Read the model definition and answer for the solid it produces. Units are mm, in the model's axes. A direction names the side the tool comes from. Give positions to 0.01 mm unless a question says otherwise; leave off trailing zeros. Write each loop counter-clockwise with the first axis right and the second up, starting at its lowest first coordinate (ties: lowest second). Pieces come first, ordered by that corner, then holes. Notation, with made-up numbers: (-12, -30) -> (-5, -30) arc R17 ccw to (-5, -5) -> close; hole circle Ø9 at (-12, -37). An arc over 180 degrees is marked (long way). Write item = value, one per line.
from build123d import *

# Parameters (mm, degrees)
SKETCH1_W           = 82.927984002
SKETCH1_H           = 60.776462656
BOSS_EXTRUDE1_DEPTH = 2
SKETCH2_W           = 82.927984002
SKETCH2_H           = 1.944543981
BOSS_EXTRUDE2_DEPTH = 55
SKETCH3_W           = 82.927984002
SKETCH3_H           = 1.52283727
BOSS_EXTRUDE3_DEPTH = 55
SKETCH4_W           = 1.238263506
SKETCH4_H           = 57.309081405
BOSS_EXTRUDE4_DEPTH = 55
SKETCH5_W           = 55
SKETCH5_H           = 1.968247646
BOSS_EXTRUDE5_DEPTH = 59
SKETCH6_W           = 41.500434797
SKETCH6_H           = 30.602093287
CUT_EXTRUDE1_DEPTH  = 59


with BuildPart() as part:
    # Sketch1 → Boss-Extrude1 (new body)
    with BuildSketch(Plane(origin=(0, 0, 0), x_dir=(0, 0, -1), z_dir=(1, 0, 0))):
        with Locations((-67.649308223, 21.107365524)):
            Rectangle(SKETCH1_W, SKETCH1_H)
    extrude(amount=BOSS_EXTRUDE1_DEPTH)

    # Sketch2 → Boss-Extrude2 (add)
    with BuildSketch(Plane(origin=(2, 0, 0), x_dir=(0, 0, -1), z_dir=(1, 0, 0))):
        with Locations((-67.649308223, 50.523324862)):
            Rectangle(SKETCH2_W, SKETCH2_H)
    extrude(amount=BOSS_EXTRUDE2_DEPTH)

    # Sketch3 → Boss-Extrude3 (add)
    with BuildSketch(Plane(origin=(2, 0, 0), x_dir=(0, 0, -1), z_dir=(1, 0, 0))):
        with Locations((-67.649308223, -8.519447169)):
            Rectangle(SKETCH3_W, SKETCH3_H)
    extrude(amount=BOSS_EXTRUDE3_DEPTH)

    # Sketch4 → Boss-Extrude4 (add)
    with BuildSketch(Plane(origin=(2, 0, 0), x_dir=(0, 0, -1), z_dir=(1, 0, 0))):
        with Locations((-108.494168471, 20.896512169)):
            Rectangle(SKETCH4_W, SKETCH4_H)
    extrude(amount=BOSS_EXTRUDE4_DEPTH)

    # Sketch5 → Boss-Extrude5 (add)
    with BuildSketch(Plane(origin=(0, 49.551052871, 0), x_dir=(-1, 0, 0), z_dir=(0, -1, 0))):
        with Locations((-29.5, -27.169440045)):
            Rectangle(SKETCH5_W, SKETCH5_H)
    extrude(amount=BOSS_EXTRUDE5_DEPTH)

    # Sketch6 → Cut-Extrude1 (cut)
    with BuildSketch(Plane.ZY):
        with Locations((77.408781478, 14.741773436)):
            Rectangle(SKETCH6_W, SKETCH6_H)
    extrude(amount=-CUT_EXTRUDE1_DEPTH, mode=Mode.SUBTRACT)


solid = part.part
(1) Given P1, Ø1, axis at x = 1.5, z = 68, coming from the -Y side, flat-ended and moving along its own axis, determine where the tip first touches the part or whether it passes through.
Checks:
P1 = -9.28
(2) Consider L1, parallel to Z at x = 19, y = 10; L2, parallel to Y at x = 36.5, z = 50.5; L3, parallel to X at y = 13.5, z = 36. Determine where each line is inside the solid, lowest interval first.
Checks:
L1 = 26.19 to 28.15, 107.88 to 109.11
L2 = -9.28 to -7.76, 49.55 to 51.5
L3 = 0 to 2
(3) For a pull along Z with two mould halves and no side action, classify faces 1 (the flat face through (1, 15, 98.159)), 2 (the flat face through (30, -9.449, 27)), 3 (the flat face through (29, 20, 107.875)), 4 (the flat face through (28, 21, 109.113)) as released by +Z, released by -Z, zero draft, split by the parting line, or undercut.
Checks:
face_1 = undercut
face_2 = zero draft
face_3 = undercut
face_4 = released by +Z
(4) The part is cut by section A-A on x = 53. Determine the outline of the cut face in (y, z).
Checks:
outline = (-9.45, 26.19) -> (51.5, 26.19) -> (51.5, 109.11) -> (-9.28, 109.11) -> (-9.28, 28.15) -> (-9.45, 28.15) -> close; hole (-7.76, 28.15) -> (49.55, 28.15) -> (49.55, 107.88) -> (-7.76, 107.88) -> close
(5) The part is cut by section B-B on y = 3.5. Determine the outline of the cut face in (x, z), plus the area to 3 significant figures.
Checks:
outline = (0, 26.19) -> (57, 26.19) -> (57, 28.15) -> (2, 28.15) -> (2, 56.66) -> (0, 56.66) -> close; (0, 98.16) -> (2, 98.16) -> (2, 107.88) -> (57, 107.88) -> (57, 109.11) -> (0, 109.11) -> close
area = 259 mm²
(6) The part is cut by section D-D on y = 31. Determine the outline of the cut face in (x, z).
Checks:
outline = (0, 26.19) -> (57, 26.19) -> (57, 28.15) -> (2, 28.15) -> (2, 107.88) -> (57, 107.88) -> (57, 109.11) -> (0, 109.11) -> close
(7) The part is cut by section C-C on z = 88. Determine the outline of the cut face in (x, y).
Checks:
outline = (0, -9.28) -> (57, -9.28) -> (57, -7.76) -> (2, -7.76) -> (2, -0.56) -> (0, -0.56) -> close; (0, 30.04) -> (2, 30.04) -> (2, 49.55) -> (57, 49.55) -> (57, 51.5) -> (0, 51.5) -> close
(8) A tool of negligible diameter and unlimited length cuts with its end or side. For faces 5 (the flat face through (29, 49.551, 69)), 6 (the flat face through (1, -0.559, 77)), 7 (the flat face through (57, 21, 28)), from which of +Z, -Z, +X, -X, +Y, -Y can it reach the whole face along a straight path? Write none if from no direction.
Checks:
face_5 = +X
face_6 = +X, -X
face_7 = +Z, -Z, +X, +Y, -Y
